from build123d import *

# Parameters (mm, degrees)
SKETCH_1_R         = 13.2
EXTRUDE_1_DEPTH    = 20
SKETCH1_R          = 1.5
CUT_EXTRUDE1_DEPTH = 64.415064914


with BuildPart() as part:
    # 草图1 → 凸台-拉伸1 (new body)
    with BuildSketch(Plane.XY):
        with BuildLine():
            Line((-26.636659375, 37.991533435), (-33.982028451, 20.754703285))
            ThreePointArc((-33.982028451, 20.754703285), (-20.752268235, -3.895931787), (6.444792613, 2.661525501))
            Line((6.444792613, 2.661525501), (10.6520193, 9.103214753))
            Line((10.6520193, 9.103214753), (8.9820702, 34.644311807))
            ThreePointArc((8.9820702, 34.644311807), (-2.647754906, 40.666580897), (-12.360428284, 49.452053726))
            Line((-12.360428284, 49.452053726), (-12.882509975, 49.032942563))
            Line((-12.882509975, 49.032942563), (-26.636659375, 37.991533435))
        make_face()
        with Locations((-11.400988001, 16.998271389)):
            Circle(SKETCH_1_R, mode=Mode.SUBTRACT)
    extrude(amount=EXTRUDE_1_DEPTH)

    # Sketch1 → Cut-Extrude1 (cut, through all)
    with BuildSketch(Plane(origin=(0, 0, 0), x_dir=(-1, 0, 0), z_dir=(0, 0, -1))):
        with Locations((-3.729872433, 30.054548194)):
            Circle(SKETCH1_R)
        with Locations((-311.403264346, -148.702528504)):
            Circle(SKETCH1_R)
        with Locations((18.975895674, 36.756893457)):
            Circle(SKETCH1_R)
        with Locations((29.72343959, 12.005147937)):
            Circle(SKETCH1_R)
        with Locations((0, 2.339279114)):
            Circle(SKETCH1_R)
    extrude(amount=-CUT_EXTRUDE1_DEPTH, mode=Mode.SUBTRACT)


solid = part.part
Work out the finished part from the listing and answer in its coordinate system (mm). Coordinates: 2 decimals unless noted, no trailing zeros. Write each loop counter-clockwise with the first axis right and the second up, starting at its lowest first coordinate (ties: lowest second). Pieces come first, ordered by that corner, then holes.
1. Flat-ended cylindrical pins translate along their axes: pin 1 (1.8 mm diameter, centred on x = -29.72, y = 12.01, fed in from +Z); pin 2 (3 mm diameter, centred on x = -28, z = 8, fed in from +Y); pin 3 (8 mm diameter, centred on x = -1.5, z = 6, fed in from -Y); pin 4 (12 mm diameter, centred on y = 15.5, z = 6, fed in from -X). Find the tip coordinate at first contact, or state that the pin passes through.
Results list:
pin 1: passes through
pin 2: stops at y = 38.1
pin 3: stops at y = -5.12
pin 4: stops at x = -34.29
2. The part is cut by section B-B, the plane x = -5. Write down the section's boundary in (y, z).
Results list:
outline: (-4.98, 0) - (5.45, 0) - (5.45, 20) - (-4.98, 20) - close; (28.54, 0) - (42.4, 0) - (42.4, 20) - (28.54, 20) - close
3. Consider line 1 along Y through (x, z) = (-18, 11.5); line 2 along X through (y, z) = (14, 12); line 3 along Y through (x, z) = (-21, 13.5). Determine where each line is inside the solid, lowest interval first.
Results list:
line 1: y = -4.92 to 5.57, 28.43 to 35.62, 37.9 to 44.92
line 2: x = -34.1 to -24.26, 1.45 to 10.33
line 3: y = -3.78 to 7.94, 26.06 to 42.52
4. The part is cut by section D-D, the plane x = -29.5. Write down the section's boundary in (y, z), and give its area (3 significant figures).
Results list:
outline: (2.98, 0) - (10.52, 0) - (10.52, 20) - (2.98, 20) - close; (13.49, 0) - (31.27, 0) - (31.27, 20) - (13.49, 20) - close
area: 506 mm2
5. For a pull along Y with two mould halves and no side action, classify faces 1 (the cylindrical face through (4.1, 28.6, 9.9)), 2 (the cylindrical face through (-18.781, 38.244, 9.86)), 3 (the flat face through (8.52, 5.84, 9.86)), 4 (the flat face through (-30.26, 29.49, 9.86)) as +Y half, -Y half, draft (parallel to the pull), parting line (faces both ways), or undercut.
Results list:
face 1: undercut
face 2: undercut
face 3: -Y half
face 4: +Y half
6. The part is cut by section A-A, the plane x = 0. Write down the section's boundary in (y, z), and give its area (3 significant figures).
Results list:
outline: (-2.85, 0) - (0.84, 0) - (0.84, 20) - (-2.85, 20) - close; (3.84, 0) - (10.35, 0) - (10.35, 20) - (3.84, 20) - close; (23.65, 0) - (38.95, 0) - (38.95, 20) - (23.65, 20) - close
area: 510 mm2
7. The part is cut by section C-C, the plane z = 13.5. Write down the section's boundary in (x, y), and give its area (3 significant figures).
Results list:
outline: (-33.98, 20.75) arc R22.89 ccw to (6.44, 2.66) - (10.65, 9.1) - (8.98, 34.64) arc R51 cw to (-12.36, 49.45) - (-26.64, 37.99) - close; hole circle Ø3 at (-29.72, 12.01); hole circle Ø26.4 at (-11.4, 17); hole circle Ø3 at (-18.98, 36.76); hole circle Ø3 at (0, 2.34); hole circle Ø3 at (3.73, 30.05)
area: 1,230 mm2
